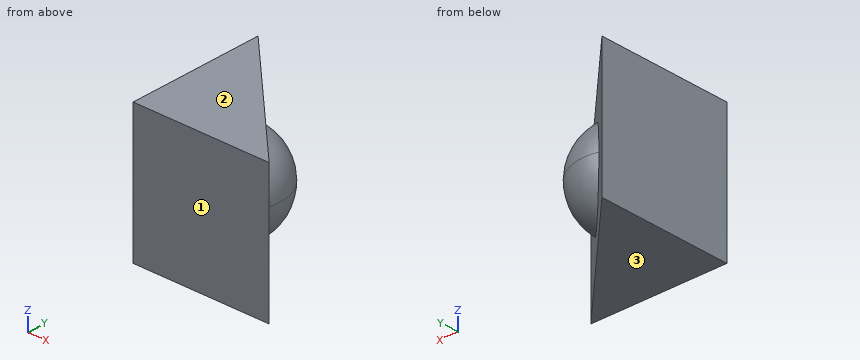
```python
from build123d import *
from build123d.topology import SkipClean

# Parameters (mm, degrees)
BOSS_EXTRUDE1_DEPTH = 25


with BuildPart() as part:
    # Sketch1 → Boss-Extrude1 (new, symmetric)
    with BuildSketch(Plane.XY):
        Polygon((0, 50), (0, 0), (50, 0), align=None)
    extrude(amount=BOSS_EXTRUDE1_DEPTH, both=True)

    # Sketch2 → Revolve1 (revolve)
    with SkipClean():  # the faces are left unmerged after this step: merging them gives an invalid solid
        with BuildSketch(Plane.XY):
            with BuildLine():
                Line((5.908116908, 31.363961031), (31.363961031, 5.908116908))
                ThreePointArc((31.363961031, 5.908116908), (31.363961031, 31.363961031), (5.908116908, 31.363961031))
            make_face()
        revolve(axis=Axis((5.908116908, 31.363961031, 0), (0.7071067811865475, -0.7071067811865476, 0)))


solid = part.part
```
Geometry: final body of the model. Coordinates: model frame, mm. Face numbers are marked on the shaded views. Coordinates: 2 decimals unless noted, no trailing zeros. Order: outer loops, then holes, each group sorted by start corner. A loop starts at its lowest first (then second) coordinate and runs counter-clockwise, first axis right, second up. Notation, with made-up numbers: M 16,9.25 L 53,9.25 A35 cw 53,41.25 Z; hole C 1.25,3 d11. An arc over 180 degrees is marked long. Answer in a Markdown table with one row per item. Add a question column.
Q1. Line query: L1, parallel to X at y = 27, z = -16; L2, parallel to X at y = 31, z = 18; L3, parallel to Y at x = 7, z = -13. Output: solid intervals per line, ascending.
Q2. Mould query, pull axis Z, two halves, no side actions, for the marked faces 1, 2 and 3. Classes: released by +Z, released by -Z, zero draft, split by the parting line, or undercut.
Q3. Section query B-B on z = -19. Return the cut outline in (x, y).
Completed:
| question | item | result |
|---|---|---|
| 1 | L1 | x = 0 to 23 |
| 1 | L2 | x = 0 to 19 |
| 1 | L3 | y = 0 to 43 |
| 2 | face 1 | zero draft |
| 2 | face 2 | released by +Z |
| 2 | face 3 | released by -Z |
| 3 | outline | M 0,0 L 50,0 L 0,50 Z |
